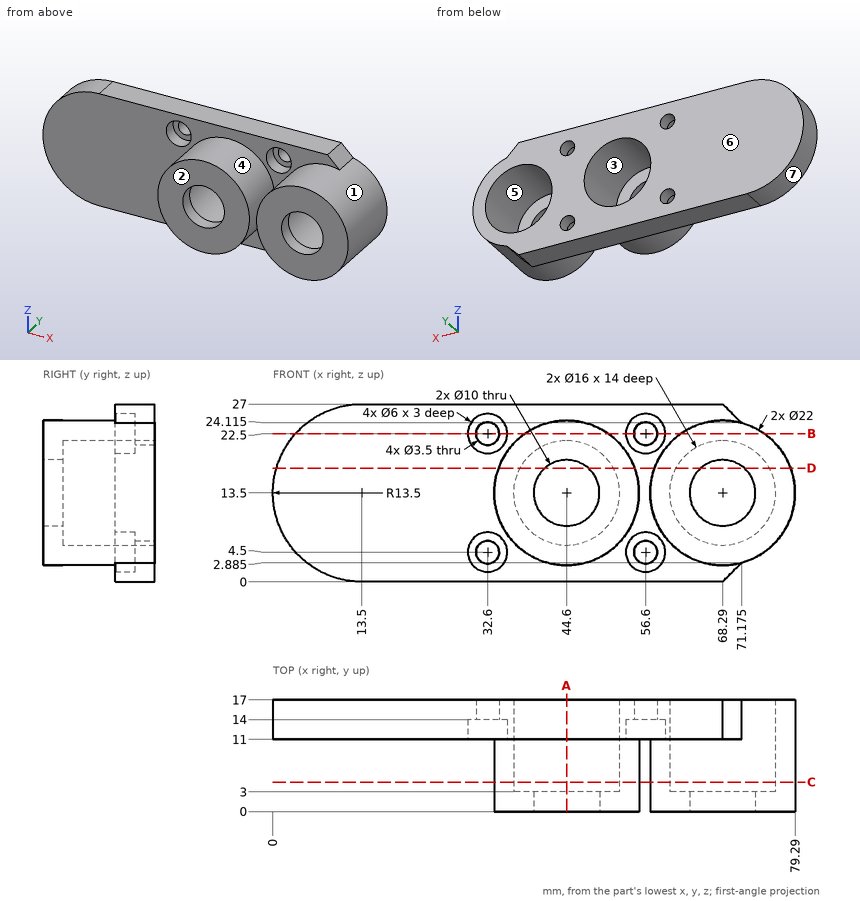
Check sheet for the drawn part. Datum: minimum x, y, z corner. Units: mm. A direction names the side the tool comes from. Give positions to 0.01 mm unless a question says otherwise; leave off trailing zeros. Loops run counter-clockwise (first coordinate to the right, second up) from the corner with the lowest first, then second, coordinate; pieces in that order, holes last.
1) Thickness scan on line 1 along X through (y, z) = (8.5, 13.5); line 2 along Z through (x, y) = (56.6, 15.35); line 3 along X through (y, z) = (1.5, 14) (1 decimal). Record the ranges inside material, lowest first.
2) Sectioned sample at D-D, the plane z = 17.25. Enter the section's corners in (x, y), then the cut area to 3 significant figures.
3) Sectioned sample at A-A, the plane x = 44.6. Enter the section's corners in (y, z).
4) Sectioned sample at B-B, the plane z = 22.5. Enter the section's corners in (x, y), then the cut area to 3 significant figures.
5) Depth check by flat-ended pin: pin 1 Ø3 at (x, z) = (33.5, 21.5) entering from -Y; pin 2 Ø13 at (x, z) = (68.29, 13.5) entering from +Y; pin 3 Ø3 at (y, z) = (7, 6) entering from -X. Enter the tip coordinate at first touch or a pass-through.
6) Sectioned sample at C-C, the plane y = 4.5. Enter the section's corners in (x, z), then the cut area to 3 significant figures.
7) Set-up check for the marked faces 1, 2 and 3: record each of +Z, -Z, +X, -X, +Y, -Y from which the full face is reachable in a straight line by a thin tool's end or side.
8) Draft check along X on the marked faces 4, 5, 6 and 7. Enter one of: pulls with the +X half, pulls with the -X half, needs draft (parallel to the pull), parting line crosses it, or undercut.
Answers:
1. line 1: x = 33.6 to 36.6, 52.6 to 55.6, 57.29 to 60.29, 76.29 to 79.29
1. line 2: z = 0 to 2.75, 6.25 to 20.75, 24.25 to 27
1. line 3: x = 33.6 to 39.6, 49.6 to 55.6, 57.3 to 63.3, 73.3 to 79.3
2. outline: (0.53, 11) - (34.26, 11) - (34.26, 0) - (41.29, 0) - (41.29, 3) - (37.53, 3) - (37.53, 17) - (0.53, 17) - close; (47.91, 0) - (54.94, 0) - (54.94, 11) - (57.95, 11) - (57.95, 0) - (64.98, 0) - (64.98, 3) - (61.22, 3) - (61.22, 17) - (51.67, 17) - (51.67, 3) - (47.91, 3) - close; (71.6, 0) - (78.63, 0) - (78.63, 17) - (75.36, 17) - (75.36, 3) - (71.6, 3) - close
2. area: 488 mm2
3. outline: (0, 2.5) - (11, 2.5) - (11, 0) - (17, 0) - (17, 5.5) - (3, 5.5) - (3, 8.5) - (0, 8.5) - close; (0, 18.5) - (3, 18.5) - (3, 21.5) - (17, 21.5) - (17, 27) - (11, 27) - (11, 24.5) - (0, 24.5) - close
4. outline: (3.44, 11) - (29.6, 11) - (29.6, 14) - (30.85, 14) - (30.85, 17) - (3.44, 17) - close; (34.35, 14) - (35.6, 14) - (35.6, 11) - (38.28, 11) - (38.28, 0) - (50.92, 0) - (50.92, 11) - (53.6, 11) - (53.6, 14) - (54.85, 14) - (54.85, 17) - (34.35, 17) - close; (58.35, 14) - (59.6, 14) - (59.6, 11) - (61.97, 11) - (61.97, 0) - (74.61, 0) - (74.61, 17) - (58.35, 17) - close
4. area: 648 mm2
5. pin 1: stops at y = 14
5. pin 2: stops at y = 3
5. pin 3: stops at x = 35.38
6. outline: circle Ø22 at (44.6, 13.5); circle Ø22 at (68.29, 13.5); hole circle Ø16 at (44.6, 13.5); hole circle Ø16 at (68.29, 13.5)
6. area: 358 mm2
7. face 1: -Y
7. face 2: +Z, -Z, +X, -X, -Y
7. face 3: +Y
8. face 4: undercut
8. face 5: undercut
8. face 6: needs draft
8. face 7: pulls with the -X half
